Source: CAD feature listing. Evaluate the final solid. Frame: model axes, mm. Give positions to 0.01 mm unless a question says otherwise; leave off trailing zeros. Order: outer loops, then holes, each group sorted by start corner. A loop starts at its lowest first (then second) coordinate and runs counter-clockwise, first axis right, second up. Notation, with made-up numbers: M 6,54.5 L 52,54.5 A17 cw 52,67.5 Z; hole C -29,79.5 d9. An arc over 180 degrees is marked long. Use CSV: the item, a comma, the result in double quotes. Start each with the question number.
1. Pin query (flat end, axial travel): P1, Ø4, axis at y = 5, z = -43, coming from the -X side; P2, Ø3, axis at y = 4, z = 17.5, coming from the +X side; P3, Ø2, axis at x = -67, y = 5, coming from the +Z side. Return the tip coordinate at first contact, or that it passes through.
2. Mould query, pull axis X, two halves, no side actions, for faces 1 (the conical face through (-83.53, 3.549, 58.453)), 2 (the conical face through (82.044, 3.549, 54.732)), 3 (the flat face through (-1, 7, 12)). Classes: released by +X, released by -X, zero draft, split by the parting line, or undercut.
3. Section query A-A, the plane x = -29.5. Return the cut outline in (y, z).
4. Line query: line 1 along Z through (x, y) = (4, 0.5); line 2 along X through (y, z) = (2.25, -6); line 3 along Z through (x, y) = (15.5, 6.25). Output: solid intervals per line, ascending. Write a range as [from, to].
5. Section query B-B, the plane z = -10. Return the cut outline in (x, y).
6. Section query C-C, the plane y = 1.5. Return the cut outline in (x, z), plus the area to 3 significant figures.
from build123d import *

# Parameters (mm, degrees)
SKETCH1_W           = 170
SKETCH1_H           = 120
BOSS_EXTRUDE1_DEPTH = 7
SKETCH2_W           = 72
SKETCH2_H           = 26.620567464
CUT_EXTRUDE1_DEPTH  = 7
SKETCH3_R           = 2
CUT_EXTRUDE5_DEPTH  = 7
SKETCH7_R           = 2
CUT_EXTRUDE7_DEPTH  = 10
SKETCH6_R           = 2
CUT_EXTRUDE10_DEPTH = 10
SKETCH9_R           = 2
CUT_EXTRUDE11_DEPTH = 10
FILLET1_R           = 5
DRAFT1_ANGLE        = 1


with BuildPart() as part:
    # Sketch1 → Boss-Extrude1 (new body)
    with BuildSketch(Plane(origin=(0, 0, 0), x_dir=(1, 0, 0), z_dir=(0, 1, 0))):
        Rectangle(SKETCH1_W, SKETCH1_H)
    extrude(amount=BOSS_EXTRUDE1_DEPTH)

    # Sketch2 → Cut-Extrude1 (cut)
    with BuildSketch(Plane(origin=(0, 7, 0), x_dir=(1, 0, 0), z_dir=(0, 1, 0))):
        with Locations((0, 1.926488435)):
            Rectangle(SKETCH2_W, SKETCH2_H)
    extrude(amount=-CUT_EXTRUDE1_DEPTH, mode=Mode.SUBTRACT)

    # Sketch3 → Cut-Extrude5 (cut)
    with BuildSketch(Plane(origin=(0, 7, 0), x_dir=(1, 0, 0), z_dir=(0, 1, 0))):
        with Locations(Location((-80, 55, 0), (0, 0, 270))):
            Circle(SKETCH3_R)
    extrude(amount=-CUT_EXTRUDE5_DEPTH, mode=Mode.SUBTRACT)

    # Sketch7 → Cut-Extrude7 (cut)
    with BuildSketch(Plane(origin=(0, 7, 0), x_dir=(1, 0, 0), z_dir=(0, 1, 0))):
        with Locations(Location((-80, -55, 0), (0, 0, 270))):
            Circle(SKETCH7_R)
    extrude(amount=-CUT_EXTRUDE7_DEPTH, mode=Mode.SUBTRACT)

    # Sketch6 → Cut-Extrude10 (cut)
    with BuildSketch(Plane(origin=(0, 7, 0), x_dir=(1, 0, 0), z_dir=(0, 1, 0))):
        with Locations(Location((80, 55, 0), (0, 0, 270))):
            Circle(SKETCH6_R)
    extrude(amount=-CUT_EXTRUDE10_DEPTH, mode=Mode.SUBTRACT)

    # Sketch9 → Cut-Extrude11 (cut)
    with BuildSketch(Plane(origin=(0, 7, 0), x_dir=(1, 0, 0), z_dir=(0, 1, 0))):
        with Locations(Location((80, -55, 0), (0, 0, 270))):
            Circle(SKETCH9_R)
    extrude(amount=-CUT_EXTRUDE11_DEPTH, mode=Mode.SUBTRACT)

    # Fillet1
    fillet1_edges = [part.edges().sort_by_distance(p)[0] for p in [
        (-85, 3.5, -60),
        (85, 3.5, -60),
        (85, 3.5, 60),
        (-85, 3.5, 60),
    ]]
    fillet(fillet1_edges, radius=FILLET1_R)

    # Draft1
    draft1_faces = [part.faces().sort_by_distance(p)[0] for p in [
        (-83.535533906, 3.5, 58.535533906),
        (-85, 3.5, 0),
        (-83.535533906, 3.5, -58.535533906),
        (0, 3.5, -60),
        (83.535533906, 3.5, -58.535533906),
        (85, 3.5, 0),
        (83.535533906, 3.5, 58.535533906),
        (0, 3.5, 60),
        (-80, 3.5, 53),
        (80, 3.5, 53),
        (80, 3.5, -57),
        (-80, 3.5, -57),
        (-36, 3.5, -1.926488435),
        (0, 3.5, -15.236772167),
        (36, 3.5, -1.926488435),
        (0, 3.5, 11.383795297),
    ]]
    draft(draft1_faces, Plane.ZX, DRAFT1_ANGLE)


solid = part.part
Result set:
1,P1,"x = -84.95"
1,P2,"x = 84.96"
1,P3,"z = 59.93"
2,face 1,"released by -X"
2,face 2,"undercut"
2,face 3,"zero draft"
3,outline,"M 0,-60 L 7,-59.88 L 7,-15.36 L 0,-15.24 Z; M 0,11.38 L 7,11.51 L 7,59.88 L 0,60 Z"
4,line 1,"[-59.99, -15.25], [11.39, 59.99]"
4,line 2,"[-84.96, -36.04], [36.04, 84.96]"
4,line 3,"[-59.89, -15.35], [11.49, 59.89]"
5,outline,"M -85,0 L -36,0 L -36.12,7 L -84.88,7 Z; M 36,0 L 85,0 L 84.88,7 L 36.12,7 Z"
6,outline,"M -84.97,-55 A4.97 ccw -80,-59.97 L 80,-59.97 A4.97 ccw 84.97,-55 L 84.97,55 A4.97 ccw 80,59.97 L -80,59.97 A4.97 ccw -84.97,55 Z; hole C -80,-55 d4.05; hole C -80,55 d4.05; hole M -36.03,-15.26 L 36.03,-15.26 L 36.03,11.41 L -36.03,11.41 Z; hole C 80,-55 d4.05; hole C 80,55 d4.05"
6,area,"18,400 mm2"
